Read the model definition and answer for the solid it produces. Units are mm, in the model's axes. Face numbers are marked on the shaded views. A direction names the side the tool comes from. Coordinates: 2 decimals unless noted, no trailing zeros. Loops run counter-clockwise (first coordinate to the right, second up) from the corner with the lowest first, then second, coordinate; pieces in that order, holes last. Notation, with made-up numbers: (38, -26) -> (73, -26) arc R21 ccw to (73, -4) -> close; hole circle Ø10 at (22.5, 27.25). An arc over 180 degrees is marked (long way). Answer as a JSON object with one key per item and string values. Group by question number.
1) Section D-D, the plane z = -0.3 is taken. Give the vertices of the cut face in (x, y).
2) Which of the six approach directions +Z, -Z, +X, -X, +Y, -Y give full straight-line access (tool end or side, diameter ignored) to the marked faces 1 and 2?
3) Section C-C, the plane y = 34 is taken. Give the vertices of the cut face in (x, z).
4) Section A-A, the plane y = 69 is taken. Give the vertices of the cut face in (x, z), plus the area to 3 significant figures.
5) Flat-ended cylindrical pins translate along their axes: P1, Ø12, axis at x = 122.5, y = 59, coming from the -Z side; P2, Ø0.5, axis at y = 31.5, z = -0.5, coming from the -X side. Find the tip coordinate at first contact, or state that the pin passes through.
6) Consider probe 1 along X at (y, z) = (72, 0.05); probe 2 along Z at (x, y) = (50.5, 54.5); probe 3 along X at (y, z) = (7, -0.45). Determine where each line is inside the solid, lowest interval first. Write a range as [from, to].
7) Section B-B, the plane x = 29.5 is taken. Give the vertices of the cut face in (y, z).
Autodesk Inventor part; units mm, degrees
ref_plane "YZ Plane" through (0, 0, 0) normal (1, 0, 0) x (0, 1, 0)
ref_plane "XZ Plane" through (0, 0, 0) normal (0, 1, 0) x (-1, 0, 0)
ref_plane "XY Plane" through (0, 0, 0) normal (0, 0, 1) x (1, 0, 0)
sketch "Sketch1" plane through (0, 0, 0) normal (0, 0, 1) x (1, 0, 0)
  line L0 (0, 0) -> (154.94, 0)
  line L1 (154.94, 0) -> (154.94, 76.2)
  line L2 (154.94, 76.2) -> (0, 76.2)
  line L3 (0, 76.2) -> (0, 0)
  dimension "d0" = 76.2
  dimension "d1" = 154.94
extrude "Extrusion1" add sketch "Sketch1" along normal blind 0.254
sketch "Sketch2" plane through (0, 0, 0.254) normal (0, 0, 1) x (1, 0, 0)
  line L0 (149.86, 73.66) -> (152.4, 73.66)
  line L1 (152.4, 73.66) -> (152.4, 62.5348)
  line L2 (152.4, 62.5348) -> (149.86, 62.5348)
  line L3 (149.86, 62.5348) -> (149.86, 73.66)
  line L4 (149.86, 13.6652) -> (152.4, 13.6652)
  line L5 (152.4, 13.6652) -> (152.4, 2.54)
  line L6 (152.4, 2.54) -> (149.86, 2.54)
  line L7 (149.86, 2.54) -> (149.86, 13.6652)
  line L8 (154.94, 0) -> (154.94, 76.2)
  line L9 (154.94, 76.2) -> (0, 76.2)
  line L10 (0, 0) -> (154.94, 0)
  point P0 (151.13, 73.66)
  point P1 (151.13, 2.54)
  dimension "d4" = 11.1252
  dimension "d5" = 2.54
  dimension "d6" = 2.54
  dimension "d7" = 2.54
  dimension "d8" = 2.54
  dimension "d9" = 11.1252
extrude "Extrusion2" cut sketch "Sketch2" against normal blind 25.4
sketch "Sketch3" plane through (154.94, 0, 0) normal (1, 0, 0) x (0, 0, -1)
  line L0 (-0.254, 76.2) -> (-0.254, 0)
  line L1 (-0.254, 76.2) -> (1.016, 76.2)
  line L2 (1.016, 76.2) -> (1.016, 0)
  line L3 (1.016, 0) -> (-0.254, 0)
  line L4 (-0.254, 0) -> (-0.254, 76.2)
  point P0 (0, 0)
  dimension "d12" = 1.27
extrude "Extrusion3" add sketch "Sketch3" along normal blind 0.254
sketch "Sketch4" plane through (0, 0, 0.254) normal (0, 0, 1) x (1, 0, 0)
  line L0 (149.86, 43.18) -> (25.4, 43.18)
  line L1 (25.4, 43.18) -> (25.4, 30.48)
  line L2 (25.4, 30.48) -> (149.86, 30.48)
  line L3 (149.86, 30.48) -> (149.86, 43.18)
  line L4 (149.86, 62.5348) -> (149.86, 73.66)
  line L5 (0, 76.2) -> (155.194, 76.2)
  line L6 (0, 76.2) -> (0, 0)
  dimension "d15" = 12.7
  dimension "d16" = 0
  dimension "d17" = 33.02
  dimension "d18" = 25.4
extrude "Extrusion4" cut sketch "Sketch4" against normal blind 25.4
properties part number "Front Back side"
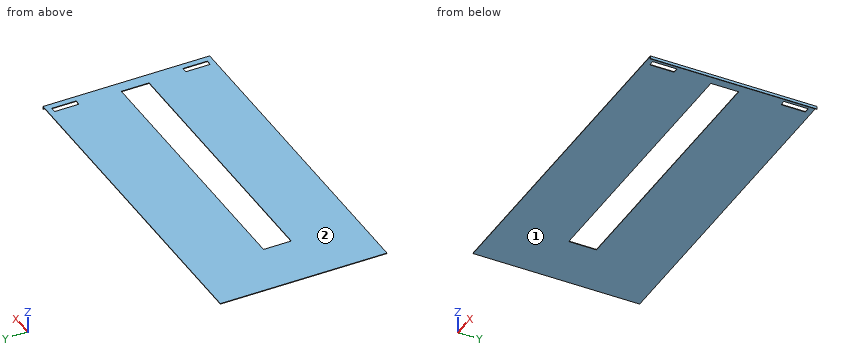
Determined:
{
 "1": {"outline": "(154.94, 0) -> (155.19, 0) -> (155.19, 76.2) -> (154.94, 76.2) -> close"},
 "2": {"face 1": "-Z, -X, +Y, -Y", "face 2": "+Z, +X, -X, +Y, -Y"},
 "3": {"outline": "(0, 0) -> (25.4, 0) -> (25.4, 0.25) -> (0, 0.25) -> close; (149.86, 0) -> (154.94, 0) -> (154.94, -1.02) -> (155.19, -1.02) -> (155.19, 0.25) -> (149.86, 0.25) -> close"},
 "4": {"outline": "(0, 0) -> (149.86, 0) -> (149.86, 0.25) -> (0, 0.25) -> close; (152.4, 0) -> (154.94, 0) -> (154.94, -1.02) -> (155.19, -1.02) -> (155.19, 0.25) -> (152.4, 0.25) -> close", "area": "39.0 mm²"},
 "5": {"P1": "z = 0", "P2": "x = 154.94"},
 "6": {"probe 1": "[0, 149.86], [152.4, 155.19]", "probe 2": "[0, 0.25]", "probe 3": "[154.94, 155.19]"},
 "7": {"outline": "(0, 0) -> (30.48, 0) -> (30.48, 0.25) -> (0, 0.25) -> close; (43.18, 0) -> (76.2, 0) -> (76.2, 0.25) -> (43.18, 0.25) -> close"}
}
